Check sheet for the modelled part. Datum: model origin and axes. Units: mm. Face numbers are marked on the shaded views. A direction names the side the tool comes from. Round coordinates to 2 decimals unless told otherwise and drop trailing zeros. Loops run counter-clockwise (first coordinate to the right, second up) from the corner with the lowest first, then second, coordinate; pieces in that order, holes last. Notation, with made-up numbers: (-34.75, 67) -> (0.25, 67) arc R32 ccw to (0.25, 105) -> close; hole circle Ø4 at (25, 53.25). An arc over 180 degrees is marked (long way). One line per item, written item: value. Start each with the question number.
1. Material ranges on L1, parallel to Y at x = 0, z = 107.95; L2, parallel to Z at x = 2.75, y = 4; L3, parallel to X at y = 4.75, z = 34.5, recorded low to high.
2. Cross-section at A-A on z = 62. Record the cut outline in (x, y), then the cut area to 3 significant figures.
3. Set-up check for the marked faces 1 and 2: record each of +Z, -Z, +X, -X, +Y, -Y from which the full face is reachable in a straight line by a thin tool's end or side.
4. Go/stop test with flat-tipped pins: pin 1 (8 mm diameter, centred on x = -8.5, y = 3, fed in from -Z); pin 2 (1 mm diameter, centred on x = -3.5, z = 25, fed in from +Y); pin 3 (2 mm diameter, centred on y = 0, z = 31.5, fed in from +X). Record where each tip stops, or that it passes through.
from build123d import *

# Parameters (mm, degrees)
SKETCH1_R           = 5.45
BOSS_EXTRUDE1_DEPTH = 110
SKETCH6_R           = 2.5
BOSS_EXTRUDE2_DEPTH = 2.5
SKETCH7_R           = 2.65
CUT_EXTRUDE1_DEPTH  = 3
JOIN1_START         = 50
JOIN1_DEPTH         = 5


# Read off the part's stored shape, not the designer's step: Join1
with BuildPart() as part:
    # Sketch1 → Boss-Extrude1 (new body)
    with BuildSketch(Plane.XY):
        Circle(SKETCH1_R)
    extrude(amount=BOSS_EXTRUDE1_DEPTH)

    # Sketch6 → Boss-Extrude2 (add)
    with BuildSketch(Plane(origin=(0, 0, 0), x_dir=(-1, 0, 0), z_dir=(0, 0, -1))):
        Circle(SKETCH6_R)
    extrude(amount=BOSS_EXTRUDE2_DEPTH)

    # Sketch7 → Cut-Extrude1 (cut)
    with BuildSketch(Plane.XY.offset(110)):
        Circle(SKETCH7_R)
    extrude(amount=-CUT_EXTRUDE1_DEPTH, mode=Mode.SUBTRACT)

    # Join1 outline → Join1 (add)
    with BuildSketch(Plane.XY.offset(JOIN1_START)):
        with BuildLine():
            ThreePointArc((-9.285244381, -7.990415307), (-9.065544683, -8.238834845), (-8.839200881, -8.481216173))
            ThreePointArc((-8.839200881, -8.481216173), (-6.788114029, -7.918067874), (-5.275945069, -6.422260963))
            ThreePointArc((-5.275945069, -6.422260963), (-4.494503923, -6.991456696), (-3.652254242, -7.466061291))
            ThreePointArc((-3.652254242, -7.466061291), (-4.385263154, -9.462756364), (-4.046049861, -11.562524833))
            ThreePointArc((-4.046049861, -11.562524833), (-3.731574572, -11.667812615), (-3.414364426, -11.764549102))
            ThreePointArc((-3.414364426, -11.764549102), (-1.919645256, -10.251304943), (-1.357971977, -8.199813678))
            ThreePointArc((-1.357971977, -8.199813678), (-0.396626227, -8.30203107), (0.570085691, -8.291925865))
            ThreePointArc((0.570085691, -8.291925865), (0.933628889, -10.387618978), (2.277280452, -12.036465168))
            ThreePointArc((2.277280452, -12.036465168), (2.602267932, -11.970409417), (2.92534822, -11.895580599))
            ThreePointArc((2.92534822, -11.895580599), (3.463190913, -9.83771313), (2.923868609, -7.78023294))
            ThreePointArc((2.923868609, -7.78023294), (3.807527147, -7.388082923), (4.639671624, -6.8959756))
            ThreePointArc((4.639671624, -6.8959756), (6.002355825, -8.529127476), (7.990415307, -9.285244381))
            ThreePointArc((7.990415307, -9.285244381), (8.238834845, -9.065544683), (8.481216173, -8.839200881))
            ThreePointArc((8.481216173, -8.839200881), (7.918067874, -6.788114029), (6.422260963, -5.275945069))
            ThreePointArc((6.422260963, -5.275945069), (6.991456696, -4.494503923), (7.466061291, -3.652254242))
            ThreePointArc((7.466061291, -3.652254242), (9.462756364, -4.385263154), (11.562524833, -4.046049861))
            ThreePointArc((11.562524833, -4.046049861), (11.667812615, -3.731574572), (11.764549102, -3.414364426))
            ThreePointArc((11.764549102, -3.414364426), (10.251304943, -1.919645256), (8.199813678, -1.357971977))
            ThreePointArc((8.199813678, -1.357971977), (8.30203107, -0.396626227), (8.291925865, 0.570085691))
            ThreePointArc((8.291925865, 0.570085691), (10.387618978, 0.933628889), (12.036465168, 2.277280452))
            ThreePointArc((12.036465168, 2.277280452), (11.970409417, 2.602267932), (11.895580599, 2.92534822))
            ThreePointArc((11.895580599, 2.92534822), (9.83771313, 3.463190913), (7.78023294, 2.923868609))
            ThreePointArc((7.78023294, 2.923868609), (7.388082923, 3.807527147), (6.8959756, 4.639671624))
            ThreePointArc((6.8959756, 4.639671624), (8.529127476, 6.002355825), (9.285244381, 7.990415307))
            ThreePointArc((9.285244381, 7.990415307), (9.065544683, 8.238834845), (8.839200881, 8.481216173))
            ThreePointArc((8.839200881, 8.481216173), (6.788114029, 7.918067874), (5.275945069, 6.422260963))
            ThreePointArc((5.275945069, 6.422260963), (4.494503923, 6.991456696), (3.652254242, 7.466061291))
            ThreePointArc((3.652254242, 7.466061291), (4.385263154, 9.462756364), (4.046049861, 11.562524833))
            ThreePointArc((4.046049861, 11.562524833), (3.731574572, 11.667812615), (3.414364426, 11.764549102))
            ThreePointArc((3.414364426, 11.764549102), (1.919645256, 10.251304943), (1.357971977, 8.199813678))
            ThreePointArc((1.357971977, 8.199813678), (0.396626227, 8.30203107), (-0.570085691, 8.291925865))
            ThreePointArc((-0.570085691, 8.291925865), (-0.933628889, 10.387618978), (-2.277280452, 12.036465168))
            ThreePointArc((-2.277280452, 12.036465168), (-2.602267932, 11.970409417), (-2.92534822, 11.895580599))
            ThreePointArc((-2.92534822, 11.895580599), (-3.463190913, 9.83771313), (-2.923868609, 7.78023294))
            ThreePointArc((-2.923868609, 7.78023294), (-3.807527147, 7.388082923), (-4.639671624, 6.8959756))
            ThreePointArc((-4.639671624, 6.8959756), (-6.002355825, 8.529127476), (-7.990415307, 9.285244381))
            ThreePointArc((-7.990415307, 9.285244381), (-8.238834845, 9.065544683), (-8.481216173, 8.839200881))
            ThreePointArc((-8.481216173, 8.839200881), (-7.918067874, 6.788114029), (-6.422260963, 5.275945069))
            ThreePointArc((-6.422260963, 5.275945069), (-6.991456696, 4.494503923), (-7.466061291, 3.652254242))
            ThreePointArc((-7.466061291, 3.652254242), (-9.462756364, 4.385263154), (-11.562524833, 4.046049861))
            ThreePointArc((-11.562524833, 4.046049861), (-11.667812615, 3.731574572), (-11.764549102, 3.414364426))
            ThreePointArc((-11.764549102, 3.414364426), (-10.251304943, 1.919645256), (-8.199813678, 1.357971977))
            ThreePointArc((-8.199813678, 1.357971977), (-8.30203107, 0.396626227), (-8.291925865, -0.570085691))
            ThreePointArc((-8.291925865, -0.570085691), (-10.387618978, -0.933628889), (-12.036465168, -2.277280452))
            ThreePointArc((-12.036465168, -2.277280452), (-11.970409417, -2.602267932), (-11.895580599, -2.92534822))
            ThreePointArc((-11.895580599, -2.92534822), (-9.83771313, -3.463190913), (-7.78023294, -2.923868609))
            ThreePointArc((-7.78023294, -2.923868609), (-7.388082923, -3.807527147), (-6.8959756, -4.639671624))
            ThreePointArc((-6.8959756, -4.639671624), (-8.529127476, -6.002355825), (-9.285244381, -7.990415307))
        make_face()
    extrude(amount=JOIN1_DEPTH)


solid = part.part
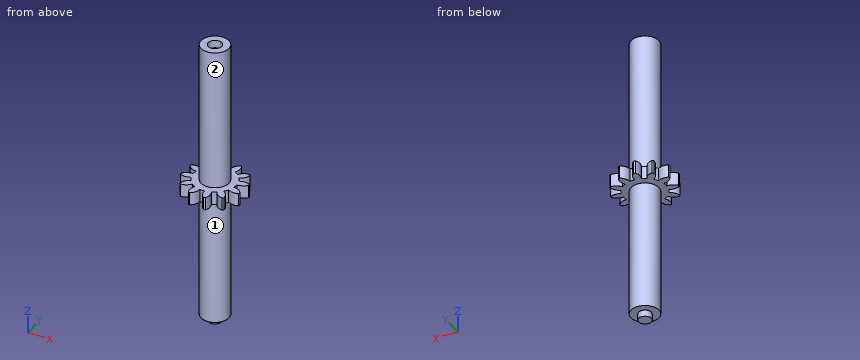
Taken from the geometry:
1. L1: y = -5.45 to -2.65, 2.65 to 5.45
1. L2: z = 0 to 110
1. L3: x = -2.67 to 2.67
2. outline: circle Ø10.9 at (0, 0)
2. area: 93.3 mm2
3. face 1: -Z
3. face 2: +Z
4. pin 1: stops at z = 0
4. pin 2: stops at y = 4.55
4. pin 3: stops at x = 5.45
